Source: CAD feature listing. Evaluate the final solid. Frame: model axes, mm. Give positions to 0.01 mm unless a question says otherwise; leave off trailing zeros. Order: outer loops, then holes, each group sorted by start corner. A loop starts at its lowest first (then second) coordinate and runs counter-clockwise, first axis right, second up. Notation, with made-up numbers: (-16.5, 17.5) - (16.5, 17.5) arc R24 ccw to (16.5, 36.5) - close; hole circle Ø9 at (21, 31). An arc over 180 degrees is marked (long way). Write each question's results on one line, items separated by ' | '. Start each with the question number.
Item 1: Contact query for flat-ended pins moving along their axis: pin 1 Ø2 at (x, z) = (-48.5, 26) entering from +Y; pin 2 Ø5 at (x, z) = (-18.5, 26.5) entering from -Y. Output: stop coordinate, or through.
Item 2: Section C-C on y = -6.5. Output: boundary loops of the cut face in (x, z).
Item 3: Section B-B on z = -28. Output: boundary loops of the cut face in (x, y), and give its area (3 significant figures).
Item 4: Section A-A on x = 47. Output: boundary loops of the cut face in (y, z), and give its area (3 significant figures).
```python
from build123d import *

# Parameters (mm, degrees)
F0_W     = 122.5050538778
F0_H     = 71.8133747578
F1_DEPTH = 33.1241749227
F2_T     = -3
F3_T     = -0.1


with BuildPart() as f1:
    # F0 (on Front) → F1 (new body)
    with BuildSketch(Plane.XZ):
        Rectangle(F0_W, F0_H)
    extrude(amount=F1_DEPTH)

    # F2
    f2_openings = [f1.faces().sort_by_distance(p)[0] for p in [
        (0, -33.124175, 0),
    ]]
    offset(amount=F2_T, openings=f2_openings)

    # F3 (hollow: no face is removed)
    offset(amount=F3_T, kind=Kind.INTERSECTION, mode=Mode.SUBTRACT)


solid = f1.part
```
Evaluation:
1) pin 1: stops at y = 0 | pin 2: stops at y = -3
2) outline: (-61.25, -35.91) - (61.25, -35.91) - (61.25, 35.91) - (-61.25, 35.91) - close; (-58.35, -33.01) - (58.35, -33.01) - (58.35, 33.01) - (-58.35, 33.01) - close; hole (-61.15, -35.81) - (61.15, -35.81) - (61.15, 35.81) - (-61.15, 35.81) - close; hole (-58.25, -32.91) - (58.25, -32.91) - (58.25, 32.91) - (-58.25, 32.91) - close
3) outline: (-61.25, -33.12) - (-58.25, -33.12) - (-58.25, -3) - (58.25, -3) - (58.25, -33.12) - (61.25, -33.12) - (61.25, 0) - (-61.25, 0) - close; hole (-61.15, -33.02) - (-58.35, -33.02) - (-58.35, -2.9) - (58.35, -2.9) - (58.35, -33.02) - (61.15, -33.02) - (61.15, -0.1) - (-61.15, -0.1) - close | area: 37.1 mm^2
4) outline: (-33.12, -35.91) - (0, -35.91) - (0, 35.91) - (-33.12, 35.91) - (-33.12, 32.91) - (-3, 32.91) - (-3, -32.91) - (-33.12, -32.91) - close; hole (-33.02, -35.81) - (-0.1, -35.81) - (-0.1, 35.81) - (-33.02, 35.81) - (-33.02, 33.01) - (-2.9, 33.01) - (-2.9, -33.01) - (-33.02, -33.01) - close | area: 27.0 mm^2
